Here's how the part is built. I have some questions about the finished solid (model axes, mm). Coordinates: 2 decimals unless noted, no trailing zeros. Loops run counter-clockwise (first coordinate to the right, second up) from the corner with the lowest first, then second, coordinate; pieces in that order, holes last.
from build123d import *

# Parameters (mm, degrees)
F1_DEPTH = 100
F2_W     = 5
F2_H     = 581
F2_W_2   = 1636.7888212204
F2_H_2   = 5
F2_W_3   = 600
F2_H_3   = 1200
F2_W_4   = 607.3750638962
F3_DEPTH = 25
F4_W     = 2650
F4_H     = 5
F5_DEPTH = 25


with BuildPart() as f1:
    # F0 (on Right) → F1 (new body)
    with BuildSketch(Plane.YZ):
        Polygon((389.0280389786, 634.7590853661), (389.0280389786, 33.4885828197), (1817.3750638962, 33.4885828197), (1817.3750638962, 1675.6669797748), align=None)
    extrude(amount=-F1_DEPTH)

    # F2 (on Right) → F3 (cut)
    with BuildSketch(Plane.YZ):
        with Locations((1214.8750638962, 1528.9885828197)):
            Rectangle(F2_W, F2_H)
        with Locations((2035.7694745064, 1235.9885828197)):
            Rectangle(F2_W_2, F2_H_2)
        with Locations((1214.8750638962, 1235.9885828197)):
            Rectangle(F2_W, F2_H_2)
        with Locations((912.3750638962, 1235.9885828197)):
            Rectangle(F2_W_3, F2_H_2)
        with Locations((1214.8750638962, 633.4885828197)):
            Rectangle(F2_W, F2_H_3)
        with Locations((609.8750638962, 1528.9885828197)):
            Rectangle(F2_W, F2_H)
        with Locations((609.8750638962, 1235.9885828197)):
            Rectangle(F2_W, F2_H_2)
        with Locations((609.8750638962, 633.4885828197)):
            Rectangle(F2_W, F2_H_3)
        with Locations((303.6875319481, 1235.9885828197)):
            Rectangle(F2_W_4, F2_H_2)
    extrude(amount=-F3_DEPTH, mode=Mode.SUBTRACT)

    # F4 (on face) → F5 (cut)
    with BuildSketch(Plane.YZ):
        with Locations((1624.0280389786, 785.9885828197)):
            Rectangle(F4_W, F4_H)
    extrude(amount=-F5_DEPTH, mode=Mode.SUBTRACT)


solid = f1.part
Q1. Suppose I cut it at B-B on z = 1066. Write out the boundary of the cut face in (x, y), and give its area (3 significant figures).
Q2. Please list where these lines run through material, in increasing order: probe 1 along Y at (x, z) = (-16, 560); probe 2 along Y at (x, z) = (-13.5, 1150); probe 3 along Z at (x, y) = (-6, 725.5).
Q3. Suppose I cut it at D-D on y = 1267.5. Write out the boundary of the cut face in (x, z), and give its area (3 significant figures).
Q4. Suppose I cut it at C-C on x = -60.5. Write out the boundary of the cut face in (y, z).
Q5. Will these pins go through, and if not, where does the flat tip stop? P1, Ø12, axis at x = -45.5, y = 1672.5, coming from the +Z side; P2, Ø7, axis at x = -10.5, y = 597.5, coming from the +Z side; P3, Ø1.4, axis at x = -12, y = 1211.5, coming from the +Z side.
Q6. Suppose I cut it at A-A on y = 1097.5. Write out the boundary of the cut face in (x, z), and give its area (3 significant figures).
Check values:
1. outline: (-100, 980.78) - (0, 980.78) - (0, 1212.38) - (-25, 1212.38) - (-25, 1217.38) - (0, 1217.38) - (0, 1817.38) - (-100, 1817.38) - close
1. area: 83,500 mm2
2. probe 1: y = 389.03 to 607.38, 612.38 to 1212.38, 1217.38 to 1817.38
2. probe 2: y = 1096.05 to 1212.38, 1217.38 to 1817.38
2. probe 3: z = 33.49 to 783.49, 788.49 to 879.96
3. outline: (-100, 33.49) - (0, 33.49) - (0, 783.49) - (-25, 783.49) - (-25, 788.49) - (0, 788.49) - (0, 1233.49) - (-25, 1233.49) - (-25, 1238.49) - (0, 1238.49) - (0, 1274.95) - (-100, 1274.95) - close
3. area: 124,000 mm2
4. outline: (389.03, 33.49) - (1817.38, 33.49) - (1817.38, 1675.67) - (389.03, 634.76) - close
5. P1: stops at z = 1574.46
5. P2: stops at z = 789.23
5. P3: stops at z = 1233.49
6. outline: (-100, 33.49) - (0, 33.49) - (0, 783.49) - (-25, 783.49) - (-25, 788.49) - (0, 788.49) - (0, 1151.06) - (-100, 1151.06) - close
6. area: 112,000 mm2
